```python
from build123d import *

# Parameters (mm, degrees)
EXTRUDE_1_DEPTH     = 10
CUT_EXTRUDE_1_DEPTH = 7
CUT_EXTRUDE_2_DEPTH = 7
SKETCH_4_R          = 10
CUT_EXTRUDE_3_DEPTH = 7


with BuildPart() as part:
    # 草图1 → 凸台-拉伸1 (new body)
    with BuildSketch(Plane.XY):
        with BuildLine():
            Line((10, 108), (114, 108))
            ThreePointArc((114, 108), (121.071067812, 105.071067812), (124, 98))
            Line((124, 98), (124, 10))
            ThreePointArc((124, 10), (121.071067812, 2.928932188), (114, 0))
            Line((114, 0), (10, 0))
            ThreePointArc((10, 0), (2.928932188, 2.928932188), (0, 10))
            Line((0, 10), (0, 98))
            ThreePointArc((0, 98), (2.928932188, 105.071067812), (10, 108))
        make_face()
    extrude(amount=EXTRUDE_1_DEPTH)

    # 草图2 → 切除-拉伸1 (cut)
    with BuildSketch(Plane.XY.offset(10)):
        with BuildLine():
            Line((15, 103), (109, 103))
            ThreePointArc((109, 103), (116.071067812, 100.071067812), (119, 93))
            Line((119, 93), (119, 15))
            ThreePointArc((119, 15), (116.071067812, 7.928932188), (109, 5))
            Line((109, 5), (15, 5))
            ThreePointArc((15, 5), (7.928932188, 7.928932188), (5, 15))
            Line((5, 15), (5, 93))
            ThreePointArc((5, 93), (7.928932188, 100.071067812), (15, 103))
        make_face()
    extrude(amount=-CUT_EXTRUDE_1_DEPTH, mode=Mode.SUBTRACT)

    # 草图3 → 切除-拉伸2 (cut)
    with BuildSketch(Plane(origin=(0, 0, 0), x_dir=(-1, 0, 0), z_dir=(0, 0, -1))):
        with BuildLine():
            Line((-84, 60), (-40, 60))
            ThreePointArc((-40, 60), (-32.928932188, 57.071067812), (-30, 50))
            Line((-30, 50), (-30, 18))
            ThreePointArc((-30, 18), (-32.928932188, 10.928932188), (-40, 8))
            Line((-40, 8), (-84, 8))
            ThreePointArc((-84, 8), (-91.071067812, 10.928932188), (-94, 18))
            Line((-94, 18), (-94, 50))
            ThreePointArc((-94, 50), (-91.071067812, 57.071067812), (-84, 60))
        make_face()
    extrude(amount=-CUT_EXTRUDE_2_DEPTH, mode=Mode.SUBTRACT)

    # 草图4 → 切除-拉伸3 (cut)
    with BuildSketch(Plane(origin=(0, 0, 0), x_dir=(-1, 0, 0), z_dir=(0, 0, -1))):
        with Locations((-84, 78)):
            Circle(SKETCH_4_R)
        with Locations((-40, 78)):
            Circle(SKETCH_4_R)
    extrude(amount=-CUT_EXTRUDE_3_DEPTH, mode=Mode.SUBTRACT)


solid = part.part
```
For this review, take the finished solid that the model builds, in its own axes (mm). A direction names the side the tool comes from. Coordinates: 2 decimals unless noted, no trailing zeros. Write each loop counter-clockwise with the first axis right and the second up, starting at its lowest first coordinate (ties: lowest second). Pieces come first, ordered by that corner, then holes. Notation, with made-up numbers: (-16.5, 8.5) - (5.5, 8.5) arc R15 ccw to (5.5, 28.5) - close; hole circle Ø4 at (25.25, -35.75). An arc over 180 degrees is marked (long way). Answer in a Markdown table with one row per item. Add a question column.
Q1. For probe 1 along Y at (x, z) = (40, 2.25); probe 2 along X at (y, z) = (24, 2.25); probe 3 along X at (y, z) = (80, 9.75), list the stretches that pass through material, from the lowest coordinate up.
Q2. We need section A-A, the plane y = 46.5. State the section outline as (x, z) points, and give its area (3 significant figures).
Q3. Draft analysis for pull direction Y (two halves, no side actions). For faces 1 (the cylindrical face through (3.01, 2.85, 4.93)), 2 (the flat face through (0, 53, 5)), 3 (the flat face through (119, 55, 7)), 4 (the cylindrical face through (32.85, 11.01, 1.48)), state which applies: +Y half, -Y half, draft (parallel to the pull), parting line (faces both ways), or undercut.
Q4. We need section B-B, the plane z = 6.75. State the section outline as (x, y) points, and give its area (3 significant figures).
Q5. For P1, Ø8, axis at x = 97, y = 89, coming from the +Z side; P2, Ø1.5, axis at x = 96, y = 89, coming from the -Z side, all flat-tipped, find the tip position at first contact; note any pin that passes through.
Q6. We need section C-C, the plane y = 78. State the section outline as (x, z) points.
Q7. We need section D-D, the plane x = 101. State the section outline as (y, z) points, and give its area (3 significant figures).
Q8. Tool access review of faces 5 (the flat face through (62, 60, 1)), 6 (the flat face through (61, 103, 7)), 7 (the cylindrical face through (121.15, 3.01, 4.93)): name each direction out of +Z, -Z, +X, -X, +Y, -Y from which nothing blocks a thin tool from reaching the whole face with its end or side.
Answer list:
| question | item | result |
|---|---|---|
| 1 | probe 1 | y = 0 to 8, 60 to 68, 88 to 108 |
| 1 | probe 2 | x = 0 to 30, 94 to 124 |
| 1 | probe 3 | x = 0 to 5, 119 to 124 |
| 2 | outline | (0, 0) - (30, 0) - (30, 3) - (5, 3) - (5, 10) - (0, 10) - close; (94, 0) - (124, 0) - (124, 10) - (119, 10) - (119, 3) - (94, 3) - close |
| 2 | area | 250 mm2 |
| 3 | face 1 | -Y half |
| 3 | face 2 | draft |
| 3 | face 3 | undercut |
| 3 | face 4 | undercut |
| 4 | outline | (0, 10) arc R10 ccw to (10, 0) - (114, 0) arc R10 ccw to (124, 10) - (124, 98) arc R10 ccw to (114, 108) - (10, 108) arc R10 ccw to (0, 98) - close; hole (5, 15) arc R10 ccw to (15, 5) - (109, 5) arc R10 ccw to (119, 15) - (119, 93) arc R10 ccw to (109, 103) - (15, 103) arc R10 ccw to (5, 93) - close |
| 4 | area | 2,220 mm2 |
| 5 | P1 | stops at z = 3 |
| 5 | P2 | stops at z = 0 |
| 6 | outline | (0, 0) - (30, 0) - (30, 3) - (5, 3) - (5, 10) - (0, 10) - close; (50, 0) - (74, 0) - (74, 3) - (50, 3) - close; (94, 0) - (124, 0) - (124, 10) - (119, 10) - (119, 3) - (94, 3) - close |
| 7 | outline | (0, 0) - (108, 0) - (108, 10) - (103, 10) - (103, 3) - (5, 3) - (5, 10) - (0, 10) - close |
| 7 | area | 394 mm2 |
| 8 | face 5 | +Z, -Z |
| 8 | face 6 | +Z |
| 8 | face 7 | +Z, -Z, +X, -Y |
